```python
from build123d import *

# Parameters (mm, degrees)
SKETCH_1_W          = 164
SKETCH_1_H          = 85
EXTRUDE_1_DEPTH     = 2
SKETCH_2_R          = 1.5
CUT_EXTRUDE_1_DEPTH = 2
SKETCH_4_W          = 56
SKETCH_4_H          = 44
CUT_EXTRUDE_3_DEPTH = 10
EXTRUDE_2_DEPTH     = 2
SKETCH_9_R          = 1.5
CUT_EXTRUDE_6_DEPTH = 10
CUT_EXTRUDE_7_DEPTH = 10
CUT_EXTRUDE_8_DEPTH = 10
FILLET_3_R          = 2
FILLET_4_R          = 2


with BuildPart() as part:
    # 草图1 → 凸台-拉伸1 (new body)
    with BuildSketch(Plane(origin=(0, 0, 0), x_dir=(1, 0, 0), z_dir=(0, 1, 0))):
        Rectangle(SKETCH_1_W, SKETCH_1_H)
    extrude(amount=EXTRUDE_1_DEPTH)

    # 草图2 → 切除-拉伸1 (cut)
    with BuildSketch(Plane(origin=(0, 2, 0), x_dir=(1, 0, 0), z_dir=(0, 1, 0))):
        with Locations(Location((31, 25, 0), (0, 0, 270))):
            Circle(SKETCH_2_R)
        with Locations(Location((-31, 25, 0), (0, 0, 270))):
            Circle(SKETCH_2_R)
        with Locations(Location((-31, -25, 0), (0, 0, 270))):
            Circle(SKETCH_2_R)
        with Locations(Location((31, -25, 0), (0, 0, 270))):
            Circle(SKETCH_2_R)
    extrude(amount=-CUT_EXTRUDE_1_DEPTH, mode=Mode.SUBTRACT)

    # 草图4 → 切除-拉伸3 (cut)
    with BuildSketch(Plane(origin=(0, 2, 0), x_dir=(1, 0, 0), z_dir=(0, 1, 0))):
        Rectangle(SKETCH_4_W, SKETCH_4_H)
    extrude(amount=-CUT_EXTRUDE_3_DEPTH, mode=Mode.SUBTRACT)

    # 草图7 → 凸台-拉伸2 (add)
    with BuildSketch(Plane(origin=(0, 2, 0), x_dir=(1, 0, 0), z_dir=(0, 1, 0))):
        Polygon((0, -2.543499116), (-3.237180694, 0), (-28, -19.456500884), (-28, -22), (-24.762819306, -22), align=None)
        Polygon((0, 2.543499116), (-3.237180694, 0), (0, -2.543499116), (3.237180694, 0), align=None)
        Polygon((24.762819306, 22), (0, 2.543499116), (3.237180694, 0), (28, 19.456500884), (28, 22), align=None)
        Polygon((3.237180694, 0), (0, -2.543499116), (24.762819306, -22), (28, -22), (28, -19.456500884), align=None)
        Polygon((-28, 22), (-28, 19.456500884), (-3.237180694, 0), (0, 2.543499116), (-24.762819306, 22), align=None)
    extrude(amount=-EXTRUDE_2_DEPTH)

    # 草图9 → 切除-拉伸6 (cut)
    with BuildSketch(Plane(origin=(0, 2, 0), x_dir=(1, 0, 0), z_dir=(0, 1, 0))):
        with Locations(Location((77.5, -36.869534675, 0), (0, 0, 270))):
            Circle(SKETCH_9_R)
        with Locations(Location((77.5, 36.869534675, 0), (0, 0, 270))):
            Circle(SKETCH_9_R)
    cut_extrude_6 = extrude(amount=-CUT_EXTRUDE_6_DEPTH, mode=Mode.SUBTRACT)

    # 镜向3: 切除-拉伸6 across plane
    add(cut_extrude_6.mirror(Plane(origin=(0, 0, 0), x_dir=(0, 0, 1), z_dir=(1, 0, 0))), mode=Mode.SUBTRACT)

    # 草图11 → 切除-拉伸7 (cut)
    with BuildSketch(Plane.XZ):
        Polygon((-74.5, 33.007564849), (-34, 22.669583035), (-34, -22.669583035), (-74.5, -33.007564849), align=None)
    cut_extrude_7 = extrude(amount=-CUT_EXTRUDE_7_DEPTH, mode=Mode.SUBTRACT)

    # 镜向4: 切除-拉伸7 across plane
    add(cut_extrude_7.mirror(Plane(origin=(0, 0, 0), x_dir=(0, 0, 1), z_dir=(1, 0, 0))), mode=Mode.SUBTRACT)

    # 草图12 → 切除-拉伸8 (cut)
    with BuildSketch(Plane.XZ):
        Polygon((-79.341828688, 42.5), (-26.454329961, 29), (26.454329961, 29), (79.341828688, 42.5), align=None)
    cut_extrude_8 = extrude(amount=-CUT_EXTRUDE_8_DEPTH, mode=Mode.SUBTRACT)

    # 镜向5: 切除-拉伸8 across plane
    add(cut_extrude_8.mirror(Plane.XY), mode=Mode.SUBTRACT)

    # 圆角3
    fillet_3_edges = [part.edges().sort_by_distance(p)[0] for p in [
        (-74.5, 1, -33.007564849),
        (-74.5, 1, 33.007564849),
        (-34, 1, 22.669583035),
        (-34, 1, -22.669583035),
        (74.5, 1, 33.007564849),
        (74.5, 1, -33.007564849),
        (34, 1, -22.669583035),
        (34, 1, 22.669583035),
        (-28, 1, 19.456500884),
        (-3.237180694, 1, 0),
        (-28, 1, -19.456500884),
        (-24.762819306, 1, -22),
        (0, 1, -2.543499116),
        (24.762819306, 1, -22),
        (28, 1, -19.456500884),
        (3.237180694, 1, 0),
        (28, 1, 19.456500884),
        (24.762819306, 1, 22),
        (0, 1, 2.543499116),
        (-24.762819306, 1, 22),
    ]]
    fillet(fillet_3_edges, radius=FILLET_3_R)

    # 圆角4
    fillet_4_edges = [part.edges().sort_by_distance(p)[0] for p in [
        (-79.341828688, 1, 42.5),
        (79.341828688, 1, 42.5),
        (26.454329961, 1, 29),
        (-26.454329961, 1, 29),
        (79.341828688, 1, -42.5),
        (-79.341828688, 1, -42.5),
        (-26.454329961, 1, -29),
        (26.454329961, 1, -29),
        (82, 1, 42.5),
        (-82, 1, 42.5),
        (-82, 1, -42.5),
        (82, 1, -42.5),
    ]]
    fillet(fillet_4_edges, radius=FILLET_4_R)


solid = part.part
```
Design review of the part built by this model. Coordinates are the model's own, in mm. A direction names the side the tool comes from. Round coordinates to 2 decimals unless told otherwise and drop trailing zeros. Write each loop counter-clockwise with the first axis right and the second up, starting at its lowest first coordinate (ties: lowest second). Pieces come first, ordered by that corner, then holes. Notation, with made-up numbers: (-39.75, 56.25) -> (15.25, 56.25) arc R17 ccw to (15.25, 65.25) -> close; hole circle Ø10 at (76.5, 55.5). An arc over 180 degrees is marked (long way). Write item = value, one per line. Start each with the question number.
1) Wall thickness on probe 1 along X at (y, z) = (0.3, 12.5); probe 2 along Z at (x, y) = (77.5, 1.5); probe 3 along X at (y, z) = (1.8, -9): over which ranges is each line inside the solid? List them lowest first. Write a range as from..to.
2) Mouldability with a two-part tool opening along Z and no side actions: class faces 1 (the face through (0, 2, 0)), 2 (the face through (-54.011, 0.986, 27.778)), 3 (the face through (52.531, 0.986, -35.656)) as +Z half, -Z half, draft (parallel to the pull), parting line (faces both ways), or undercut.
3) Clearance check with flat-ended pins moving along their axes: pin 1 (0.6 mm diameter, centred on x = 5, y = 1, fed in from +Z); pin 2 (0.6 mm diameter, centred on x = -9, y = 1.5, fed in from -Z). State where each tip first meets the part, or that it passes through.
4) Take a section at C-C, the plane z = 25. State the section outline as (x, y) points, plus the area to 3 significant figures.
5) Take a section at D-D, the plane y = 0.4. Count the separate pieces of the cut face and the enclosed holes in it, plus the area to 3 significant figures.
6) Take a section at B-B, the plane x = -77.5. State the section outline as (y, z) points.
7) Take a section at A-A, the plane x = 56.5. State the section outline as (y, z) points, plus the area to 3 significant figures.
8) Tool access review of faces 4 (the face through (0, 0, 0)), 5 (the face through (-15.14, 1.01, -9.35)), 6 (the face through (-53.265, 0.986, -35.844)): name each direction out of +Z, -Z, +X, -X, +Y, -Y from which nothing blocks a thin tool from reaching the whole face with its end or side.
Results list:
q1.probe_1 = -82..-74.5, -34..-28, -19.15..-12.67, 12.67..19.15, 28..34, 74.5..82
q1.probe_2 = -42.03..-38.37, -35.37..35.37, 38.37..42.03
q1.probe_3 = -82..-74.5, -34..-28, -14.69..-8.22, 8.22..14.69, 28..34, 74.5..82
q2.face_1 = draft
q2.face_2 = undercut
q2.face_3 = -Z half
q3.pin_1 = 29
q3.pin_2 = -29
q4.outline = (-82, 0) -> (-74.5, 0) -> (-74.5, 2) -> (-82, 2) -> close; (-43.13, 0) -> (-32.5, 0) -> (-32.5, 2) -> (-43.13, 2) -> close; (-29.5, 0) -> (29.5, 0) -> (29.5, 2) -> (-29.5, 2) -> close; (32.5, 0) -> (43.13, 0) -> (43.13, 2) -> (32.5, 2) -> close; (74.5, 0) -> (82, 0) -> (82, 2) -> (74.5, 2) -> close
q4.area = 191 mm²
q5.separate_pieces = 1
q5.enclosed_holes = 14
q5.area = 4,640 mm²
q6.outline = (0, -42.03) -> (2, -42.03) -> (2, -38.37) -> (0, -38.37) -> close; (0, -35.37) -> (2, -35.37) -> (2, 35.37) -> (0, 35.37) -> close; (0, 38.37) -> (2, 38.37) -> (2, 42.03) -> (0, 42.03) -> close
q7.outline = (0, -36.67) -> (2, -36.67) -> (2, -28.41) -> (0, -28.41) -> close; (0, 28.41) -> (2, 28.41) -> (2, 36.67) -> (0, 36.67) -> close
q7.area = 33.0 mm²
q8.face_4 = +Z, -Z, +X, -X, -Y
q8.face_5 = +Y, -Y
q8.face_6 = -Z, +Y, -Y
